Verification items for this drawing (mm, ordinates from the low corner). A direction names the side the tool comes from. Coordinates: 2 decimals unless noted, no trailing zeros. Loops run counter-clockwise (first coordinate to the right, second up) from the corner with the lowest first, then second, coordinate; pieces in that order, holes last. Notation, with made-up numbers: (76.25, -18.75) -> (82.25, -18.75) arc R20 ccw to (82.25, 8.25) -> close; hole circle Ø8 at (15, 78). An arc over 180 degrees is marked (long way). Write item = value, one per line.
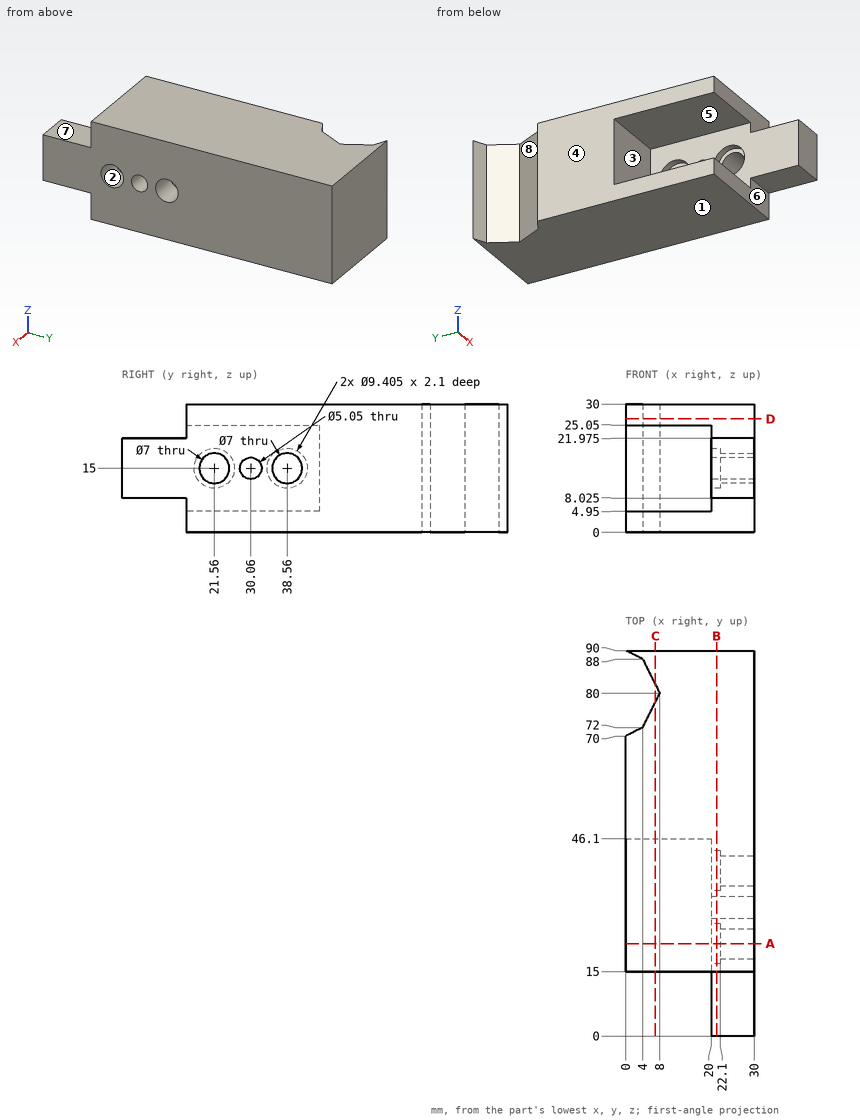
1) Release check for a two-part mould opening along Z. For the marked faces 1, 2, 3 and 4 record: pulls with the +Z half, pulls with the -Z half, needs draft (parallel to the pull), parting line crosses it, or undercut.
Ans:
face_1 = pulls with the -Z half
face_2 = undercut
face_3 = undercut
face_4 = needs draft
2) Sectioned sample at A-A, the plane y = 21.56. Record the cut outline in (x, z), plus the area to 3 significant figures.
Ans:
outline = (0, 0) -> (30, 0) -> (30, 11.5) -> (22.1, 11.5) -> (22.1, 10.3) -> (20, 10.3) -> (20, 4.95) -> (0, 4.95) -> close; (0, 25.05) -> (20, 25.05) -> (20, 19.7) -> (22.1, 19.7) -> (22.1, 18.5) -> (30, 18.5) -> (30, 30) -> (0, 30) -> close
area = 423 mm2
3) Tool access check on the marked faces 5, 6, 7 and 8. Record the directions out of +Z, -Z, +X, -X, +Y, -Y that give a thin tool (end or side, any length) a straight path to the whole face; none if there is none.
Ans:
face_5 = -X, -Y
face_6 = -Z, +X, -X, -Y
face_7 = +Z, +X, -X, -Y
face_8 = +Z, -Z, -X
4) Sectioned sample at D-D, the plane z = 26.5. Record the cut outline in (x, y).
Ans:
outline = (0, 15) -> (30, 15) -> (30, 90) -> (0, 90) -> (4, 88) -> (8, 80) -> (4, 72) -> (0, 70) -> close
5) Depth check by flat-ended pin: pin 1 Ø11 at (x, y) = (23, 6.5) entering from -Z (3 decimals); pin 2 Ø4 at (x, z) = (8, 24) entering from -Y; pin 3 Ø10 at (y, z) = (13, 16) entering from -X. Enter the tip coordinate at first touch or a pass-through.
Ans:
pin_1 = 8.025
pin_2 = 15
pin_3 = 20
6) Sectioned sample at C-C, the plane x = 7. Record the cut outline in (y, z).
Ans:
outline = (15, 0) -> (78, 0) -> (78, 30) -> (15, 30) -> (15, 25.05) -> (46.1, 25.05) -> (46.1, 4.95) -> (15, 4.95) -> close; (82, 0) -> (90, 0) -> (90, 30) -> (82, 30) -> close
7) Material ranges on line 1 (Y direction, x = 21.1, z = 15) (1 decimal); line 2 (X direction, y = 25.5, z = 19.75); line 3 (X direction, y = 40, z = 18.5), recorded low to high.
Ans:
line_1 = 0 to 16.9, 26.3 to 27.5, 32.6 to 33.9, 43.3 to 90
line_2 = 20 to 30
line_3 = 22.1 to 30
8) Sectioned sample at B-B, the plane x = 21.25. Count the separate pieces of the cut face and the enclosed holes in it, plus the area to 3 significant figures.
Ans:
separate_pieces = 1
enclosed_holes = 3
area = 2,300 mm2
